The model under review builds one solid part; all positions refer to its coordinate system, in mm. Face numbers are marked on the shaded views. A direction names the side the tool comes from. Coordinates: 2 decimals unless noted, no trailing zeros. Order: outer loops, then holes, each group sorted by start corner. A loop starts at its lowest first (then second) coordinate and runs counter-clockwise, first axis right, second up. Notation, with made-up numbers: M 10.25,62.5 L 53.25,62.5 A36 cw 53.25,99.5 Z; hole C -30,55 d2. An arc over 180 degrees is marked long. Answer in a Markdown table with one row per item.
from build123d import *

# Parameters (mm, degrees)
FILLET1_R      = 0.79375
CHAMFER1_SIZE  = 0.79375
CHAMFER1_SIZE2 = 1.374815329


with BuildPart() as part:
    # Sketch1 → Revolve1 (revolve)
    with BuildSketch(Plane.XY):
        Polygon((0, 0), (-9.398, 0), (-9.398, 1.5875), (-7.493, 4.445), (-7.493, 7.62), (-9.398, 7.62), (-9.398, 12.7), (0, 12.7), align=None)
    revolve(axis=Axis((0, 0, 0), (0, 1, 0)))

    # Fillet1
    fillet1_edges = [part.edges().sort_by_distance(p)[0] for p in [
        (9.398, 0, 0),
    ]]
    fillet(fillet1_edges, radius=FILLET1_R)

    # Chamfer1
    chamfer1_edges = [part.edges().sort_by_distance(p)[0] for p in [
        (9.398, 12.7, 0),
    ]]
    chamfer1_side = [part.faces().sort_by_distance(p)[0] for p in [
        (0, 12.7, 0),
    ]]
    chamfer(chamfer1_edges, length=CHAMFER1_SIZE, length2=CHAMFER1_SIZE2, reference=chamfer1_side[0])


solid = part.part
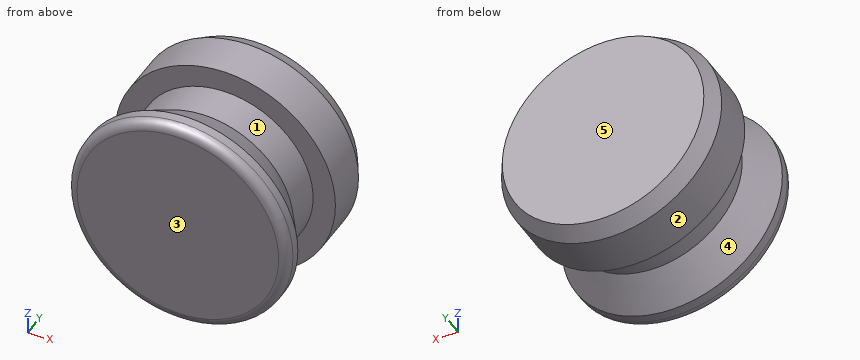
(1) Take a section at A-A (z = 0). Write out the cut boundary in (x, y) (1 decimal).
Report:
| item | result |
|---|---|
| outline | M -9.4,0.8 A0.8 ccw -8.6,0 L 8.6,0 A0.8 ccw 9.4,0.8 L 9.4,1.6 L 7.5,4.4 L 7.5,7.6 L 9.4,7.6 L 9.4,11.3 L 8.6,12.7 L -8.6,12.7 L -9.4,11.3 L -9.4,7.6 L -7.5,7.6 L -7.5,4.4 L -9.4,1.6 Z |
(2) Take a section at C-C (y = 9.5). Write out the cut boundary in (x, z).
Report:
| item | result |
|---|---|
| outline | C 0,0 d18.8 |
(3) Take a section at B-B (x = 0). Write out the cut boundary in (y, z) (1 decimal).
Report:
| item | result |
|---|---|
| outline | M 0,-8.6 A0.8 ccw 0.8,-9.4 L 1.6,-9.4 L 4.4,-7.5 L 7.6,-7.5 L 7.6,-9.4 L 11.3,-9.4 L 12.7,-8.6 L 12.7,8.6 L 11.3,9.4 L 7.6,9.4 L 7.6,7.5 L 4.4,7.5 L 1.6,9.4 L 0.8,9.4 A0.8 ccw 0,8.6 Z |
(4) Insertion check: P1, Ø4, axis at y = 6.5, z = -3, coming from the +X side; P2, Ø3, axis at y = 5.5, z = 5.5, coming from the -X side; P3, Ø2, axis at x = -1.5, y = 3.5, coming from the -Z side. Each pin has a flat end and moves straight along its axis. Give the tip position at first contact, or say it passes through.
Report:
| item | result |
|---|---|
| P1 | x = 9.3 |
| P2 | x = -6.34 |
| P3 | z = -8.68 |
(5) To check wall thickness, follow line 1 (Y direction, x = 5.5, z = -6.5); line 2 (Y direction, x = -5, z = 6); line 3 (X direction, y = 7.5, z = -0.25). State the ranges of each line that lie inside material, in increasing order. Write a range as [from, to].
Report:
| item | result |
|---|---|
| line 1 | [0, 2.91], [7.62, 12.7] |
| line 2 | [0, 3.97], [7.62, 12.7] |
| line 3 | [-7.49, 7.49] |
(6) The part is to be moulded in two halves that separate along Y. For the marked faces 3, 4 and 5, say which applies: +Y half, -Y half, draft (parallel to the pull), parting line (faces both ways), or undercut.
Report:
| item | result |
|---|---|
| face 3 | -Y half |
| face 4 | undercut |
| face 5 | +Y half |
(7) Machinability: for the marked faces 1 and 2, which of the approach directions +Z, -Z, +X, -X, +Y, -Y give a long, thin tool a straight path to every point of the face, cutting with its end or side? Answer none if there is none.
Report:
| item | result |
|---|---|
| face 1 | none |
| face 2 | +Y, -Y |
